CAD build for the part. Positions are in the model's coordinates, mm. Give positions to 0.01 mm unless a question says otherwise; leave off trailing zeros. Order: outer loops, then holes, each group sorted by start corner. A loop starts at its lowest first (then second) coordinate and runs counter-clockwise, first axis right, second up.
```python
from build123d import *

# Parameters (mm, degrees)
EXTRUDE_3_DEPTH     = 2
SKETCH_2_R          = 3.75
SKETCH_2_R_2        = 2.5
EXTRUDE_5_DEPTH     = 3
SKETCH_3_R          = 3.75
SKETCH_3_R_2        = 2.5
EXTRUDE_6_DEPTH     = 2.5
SKETCH_4_R          = 0.75
CUT_EXTRUDE_1_DEPTH = 2
SKETCH_5_R          = 2.5
EXTRUDE_7_DEPTH     = 1
SKETCH_6_R          = 2.5
CUT_EXTRUDE_2_DEPTH = 0.5
SKETCH_7_R          = 1.25
CUT_EXTRUDE_3_DEPTH = 5


with BuildPart() as part:
    # Sketch 1 → Extrude 3 (new body)
    with BuildSketch(Plane.XY):
        with BuildLine():
            Line((16.70961775, 1.988984766), (0.781737208, 3.667613248))
            ThreePointArc((0.781737208, 3.667613248), (2.914962652, 2.359129656), (3.75, 0))
            ThreePointArc((3.75, 0), (2.914962652, -2.359129656), (0.781737208, -3.667613248))
            Line((0.781737208, -3.667613248), (16.70961775, -1.988984766))
            ThreePointArc((16.70961775, -1.988984766), (18.5, 0), (16.70961775, 1.988984766))
        make_face()
    extrude(amount=EXTRUDE_3_DEPTH)



with BuildPart() as body_2:
    # Sketch 2 → Extrude 5 (new body)
    with BuildSketch(Plane.XY.offset(2)):
        Circle(SKETCH_2_R)
        Circle(SKETCH_2_R_2, mode=Mode.SUBTRACT)
    extrude(amount=EXTRUDE_5_DEPTH)


with BuildPart() as part_1:
    add(part.part)

    add(body_2.part)  # Extrude 6 merges body 2
    # Sketch 3 → Extrude 6 (add)
    with BuildSketch(Plane(origin=(0, 0, 2), x_dir=(-1, 0, 0), z_dir=(0, 0, -1))):
        Circle(SKETCH_3_R)
        Circle(SKETCH_3_R_2, mode=Mode.SUBTRACT)
    extrude(amount=EXTRUDE_6_DEPTH)

    # Sketch 4 → Cut-Extrude 1 (cut)
    with BuildSketch(Plane(origin=(0, 0, 0), x_dir=(-1, 0, 0), z_dir=(0, 0, -1))):
        with Locations((-17, 0)):
            Circle(SKETCH_4_R)
        with Locations((-7, 0)):
            Circle(SKETCH_4_R)
        with Locations((-9, 0)):
            Circle(SKETCH_4_R)
        with Locations((-11, 0)):
            Circle(SKETCH_4_R)
        with Locations((-13, 0)):
            Circle(SKETCH_4_R)
        with Locations((-15, 0)):
            Circle(SKETCH_4_R)
        with Locations((-5, 0)):
            Circle(SKETCH_4_R)
    extrude(amount=-CUT_EXTRUDE_1_DEPTH, mode=Mode.SUBTRACT)

    # Sketch 5 → Extrude 7 (add)
    with BuildSketch(Plane(origin=(0, 0, 0), x_dir=(-1, 0, 0), z_dir=(0, 0, -1))):
        Circle(SKETCH_5_R)
    extrude(amount=-EXTRUDE_7_DEPTH)

    # Sketch 6 → Cut-Extrude 2 (cut)
    with BuildSketch(Plane(origin=(0, 0, 0), x_dir=(-1, 0, 0), z_dir=(0, 0, -1))):
        Circle(SKETCH_6_R)
    extrude(amount=-CUT_EXTRUDE_2_DEPTH, mode=Mode.SUBTRACT)

    # Sketch 7 → Cut-Extrude 3 (cut)
    with BuildSketch(Plane(origin=(0, 0, 0.5), x_dir=(-1, 0, 0), z_dir=(0, 0, -1))):
        Circle(SKETCH_7_R)
    extrude(amount=-CUT_EXTRUDE_3_DEPTH, mode=Mode.SUBTRACT)


solid = part_1.part
```
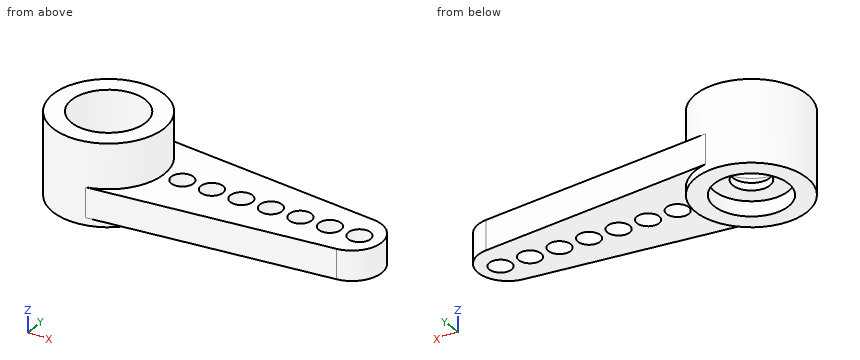
Item 1: Wall check: L1, parallel to X at y = 0, z = 3.55; L2, parallel to Z at x = 9.25, y = -1.5; L3, parallel to X at y = -1.25, z = 4.05. Give the ranges that are in metal, low to high.
Item 2: Drop flat-ended pins along their axis: pin 1 Ø2 at (y, z) = (-2, 0.5) entering from -X; pin 2 Ø2 at (x, y) = (0, 0) entering from +Z; pin 3 Ø2.5 at (x, y) = (9, 0) entering from +Z; pin 4 Ø1 at (y, z) = (0, 3) entering from +X. Give the stop position or say it passes through.
Item 3: Slice it at A-A (x = 13). Give the cut face in (y, z).
Item 4: Slice it at C-C (y = -1). Give the cut face in (x, z), and give its area (3 significant figures).
Item 5: Slice it at D-D (x = 17). Give the cut face in (y, z).
Item 6: Slice it at B-B (z = 1.3). State how many separate pieces and enclosed holes the cut face has, and give its area (3 significant figures).
A:
1. L1: x = -3.75 to -2.5, 2.5 to 3.75
1. L2: z = 0 to 2
1. L3: x = -3.54 to -2.17, 2.17 to 3.54
2. pin 1: stops at x = -3.61
2. pin 2: passes through
2. pin 3: stops at z = 2
2. pin 4: stops at x = 3.75
3. outline: (-2.38, 0) - (-0.75, 0) - (-0.75, 2) - (-2.38, 2) - close; (0.75, 0) - (2.38, 0) - (2.38, 2) - (0.75, 2) - close
4. outline: (-3.61, -0.5) - (-2.29, -0.5) - (-2.29, 0.5) - (-0.75, 0.5) - (-0.75, 1) - (-2.29, 1) - (-2.29, 5) - (-3.61, 5) - close; (0.75, 0.5) - (2.29, 0.5) - (2.29, -0.5) - (3.61, -0.5) - (3.61, 0) - (18.23, 0) - (18.23, 2) - (3.61, 2) - (3.61, 5) - (2.29, 5) - (2.29, 1) - (0.75, 1) - close
4. area: 45.3 mm2
5. outline: (-1.94, 0) - (-0.75, 0) - (-0.75, 2) - (-1.94, 2) - close; (0.75, 0) - (1.94, 0) - (1.94, 2) - (0.75, 2) - close
6. separate pieces: 1
6. enclosed holes: 8
6. area: 91.4 mm2
